Input: part model. Units: mm. Frame: model coordinates. Give positions to 0.01 mm unless a question says otherwise; leave off trailing zeros. Loops run counter-clockwise (first coordinate to the right, second up) from the corner with the lowest first, then second, coordinate; pieces in that order, holes last. Notation, with made-up numbers: (13, 68) -> (31, 68) arc R32 cw to (31, 104) -> close; hole circle Ø8 at (-32.5, 59). An arc over 180 degrees is marked (long way). Answer as a JSON object with one key per item and string values.
Autodesk Inventor part; units mm, degrees
ref_plane "YZ Plane" through (0, 0, 0) normal (1, 0, 0) x (0, 1, 0)
ref_plane "XZ Plane" through (0, 0, 0) normal (0, 1, 0) x (-1, 0, 0)
ref_plane "XY Plane" through (0, 0, 0) normal (0, 0, 1) x (1, 0, 0)
sketch "Sketch1" plane through (0, 0, 0) normal (0, 1, 0) x (-1, 0, 0)
  line L0 (37.7589, 9.4959) -> (-42.2411, 9.4959)
  line L1 (-42.2411, 9.4959) -> (-42.2411, -280.5041)
  line L2 (-42.2411, -280.5041) -> (37.7589, -280.5041)
  line L3 (27.7589, -20.5041) -> (1.7589, -20.5041)
  line L4 (1.7589, -20.5041) -> (1.7589, -65.5041)
  line L5 (1.7589, -65.5041) -> (27.7589, -65.5041)
  line L6 (27.7589, -65.5041) -> (27.7589, -20.5041)
  line L7 (-8.2411, -20.5041) -> (-34.2411, -20.5041)
  line L8 (-34.2411, -20.5041) -> (-34.2411, -65.5041)
  line L9 (-34.2411, -65.5041) -> (-8.2411, -65.5041)
  line L10 (-8.2411, -65.5041) -> (-8.2411, -20.5041)
  line L11 (-6.2411, -81.8041) -> (-32.2411, -81.8041)
  line L12 (-32.2411, -81.8041) -> (-32.2411, -156.8041)
  line L13 (-32.2411, -156.8041) -> (-6.2411, -156.8041)
  line L14 (-6.2411, -156.8041) -> (-6.2411, -81.8041)
  circle A0 centre (-3.3411, -80.5041) radius 1.5
  circle A1 centre (-34.3411, -80.5041) radius 1.5
  circle A2 centre (-3.3411, -155.5041) radius 1.5
  circle A3 centre (-34.3411, -155.5041) radius 1.5
  line L15 (37.7589, 9.4959) -> (37.7589, -280.5041)
  line L16 (37.7589, -170.5041) -> (37.7589, -280.5041)
  line L17 (12.7589, -228.5041) -> (-17.2411, -228.5041)
  line L18 (-17.2411, -228.5041) -> (-17.2411, -250.5041)
  line L19 (-17.2411, -250.5041) -> (12.7589, -250.5041)
  line L20 (12.7589, -250.5041) -> (12.7589, -228.5041)
  line L21 (12.7589, -200.5041) -> (-6.2411, -200.5041)
  line L22 (-6.2411, -200.5041) -> (-6.2411, -213.5041)
  line L23 (-6.2411, -213.5041) -> (12.7589, -213.5041)
  line L24 (12.7589, -213.5041) -> (12.7589, -200.5041)
  circle A4 centre (-7.2411, -265.5041) radius 1.5
  circle A5 centre (-7.2411, -5.5041) radius 1.5
  point P0 (0, 0)
  dimension "d0" = 290
  dimension "d1" = 80
  dimension "d4" = 45
  dimension "d5" = 26
  dimension "d6" = 30
  dimension "d8" = 45
  dimension "d9" = 26
  dimension "d10" = 30
  dimension "d11" = 10
  dimension "d12" = 75
  dimension "d13" = 26
  dimension "d16" = 1.3
  dimension "d17" = 2.9
  dimension "d18" = 3
  dimension "d20" = 31
  dimension "d22" = 3
  dimension "d23" = 75
  dimension "d24" = 3
  dimension "d25" = 75
  dimension "d26" = 3
  dimension "d27" = 15
  dimension "d28" = 10
  dimension "d32" = 22
  dimension "d33" = 30
  dimension "d34" = 25
  dimension "d35" = 30
  dimension "d36" = 13
  dimension "d37" = 19
  dimension "d38" = 25
  dimension "d39" = 15
  dimension "d40" = 45
  dimension "d41" = 15
  dimension "d42" = 3
  dimension "d43" = 45
  dimension "d44" = 15
  dimension "d45" = 3
extrude "Extrusion1" add sketch "Sketch1" along normal blind 4
sketch "Esquisse2" plane through (0, 4, 0) normal (0, 1, 0) x (1, 0, 0)
  line L0 (18.8111, 176.8041) -> (32.2411, 176.8041)
  line L1 (32.2411, 176.8041) -> (32.2411, 192.3041)
  line L2 (32.2411, 192.3041) -> (18.8111, 192.3041)
  line L3 (18.8111, 192.3041) -> (18.8111, 176.8041)
  line L4 (42.2411, -9.4959) -> (42.2411, 280.5041)
  line L5 (6.2411, 156.8041) -> (32.2411, 156.8041)
  point P0 (0, 0)
  dimension "d46" = 15.5
  dimension "d47" = 13.43
  dimension "d48" = 10
  dimension "d49" = 20
extrude "Extrusion2" cut sketch "Esquisse2" against normal through all
properties part number "support_arriere"
Q1. Ray query, line 1 along Z through (x, y) = (31.5, 2.8); line 2 along Z through (x, y) = (-12.5, 1.7); line 3 along X through (y, z) = (2.1, -31). Return the intervals inside material, ascending.
Evaluation:
{"line 1": "z = -280.5 to -192.3, -176.8 to -156.8, -81.8 to -65.5, -20.5 to 9.5", "line 2": "z = -280.5 to -250.5, -228.5 to -213.5, -200.5 to -65.5, -20.5 to 9.5", "line 3": "x = -37.76 to -27.76, -1.76 to 8.24, 34.24 to 42.24"}
Q2. Section B-B, the plane y = 2.15. Give the number of separate pieces and of enclosed holes in the cut face, then the cut area to 3 significant figures.
Evaluation:
{"separate pieces": "1", "enclosed holes": "12", "area": "17,800 mm2"}
Q3. Section A-A, the plane z = -180.5. Return the cut outline in (x, y), then the cut area to 3 significant figures.
Evaluation:
{"outline": "(-37.76, 0) -> (18.81, 0) -> (18.81, 4) -> (-37.76, 4) -> close; (32.24, 0) -> (42.24, 0) -> (42.24, 4) -> (32.24, 4) -> close", "area": "266 mm2"}
Q4. Section C-C, the plane z = -239. Return the cut outline in (x, y), then the cut area to 3 significant figures.
Evaluation:
{"outline": "(-37.76, 0) -> (-12.76, 0) -> (-12.76, 4) -> (-37.76, 4) -> close; (17.24, 0) -> (42.24, 0) -> (42.24, 4) -> (17.24, 4) -> close", "area": "200 mm2"}
